Autodesk Inventor part; units mm, degrees
ref_plane "YZ Plane" through (0, 0, 0) normal (1, 0, 0) x (0, 1, 0)
ref_plane "XZ Plane" through (0, 0, 0) normal (0, 1, 0) x (-1, 0, 0)
ref_plane "XY Plane" through (0, 0, 0) normal (0, 0, 1) x (1, 0, 0)
sketch "Sketch1" plane through (0, 0, 0) normal (1, 0, 0) x (0, 1, 0)
  line L0 (0, 0) -> (-60, 0)
  line L1 (-60, 0) -> (-60, -18)
  line L2 (-60, -18) -> (0, -18)
  line L3 (0, -18) -> (0, 0)
  line L4 (-13.5, -5.5) -> (-33.5, -5.5)
  line L5 (-37, -9) -> (-37, -9)
  line L6 (-33.5, -12.5) -> (-13.5, -12.5)
  line L7 (-10, -9) -> (-10, -9)
  arc A0 (-10, -9) -> (-13.5, -5.5) centre (-13.5, -9) ccw
  arc A1 (-13.5, -12.5) -> (-10, -9) centre (-13.5, -9) ccw
  arc A2 (-37, -9) -> (-33.5, -12.5) centre (-33.5, -9) ccw
  arc A3 (-33.5, -5.5) -> (-37, -9) centre (-33.5, -9) ccw
  point P0 (-37, -12.5)
  point P1 (-37, -5.5)
  point P2 (-10, -12.5)
  dimension "d0" = 60
  dimension "d1" = 18
  dimension "d2" = 27
  dimension "d3" = 7
  dimension "d4" = 5.5
  dimension "d5" = 10
  dimension "d6" = 3.5
extrude "Extrusion1" add sketch "Sketch1" along normal blind 3
sketch "Sketch2" plane through (3, 0, 0) normal (1, 0, 0) x (0, 0, -1)
  line L0 (18, -60) -> (18, 0)
  line L1 (0, -60) -> (18, -60)
  point P0 (0, 0)
  point P1 (9, -45)
  point P2 (9, -55)
  dimension "d9" = 9
  dimension "d10" = 9
  dimension "d11" = 5
  dimension "d12" = 10
hole "Hole1" at (3, -45, -9) at (3, -55, -9) direction (-1, 0, 0) diameter 4.4 depth 8.8 tip angle 118
fillet "Fillet1" radius 3.5 2 edges at (1.5, -60, 0) (1.5, -60, -18)
chamfer "Chamfer1" distance 0.3 angle 45 25 edges at (3, 0, -9) (3, -28.25, -18) (3, -58.9749, -16.9749) (3, -60, -9) (3, -58.9749, -1.0251) (3, -28.25, 0) (1.5, 0, -18) (0, -28.25, -18) (0, -58.9749, -16.9749) (0, -60, -9) (0, -58.9749, -1.0251) (0, -28.25, 0) (0, 0, -9) (0, -10, -9) (0, -23.5, -5.5) (0, -37, -9) (0, -23.5, -12.5) (3, -23.5, -5.5) (3, -10, -9) (3, -23.5, -12.5) (3, -37, -9) (0, -55, -6.8) (0, -45, -6.8) (3, -55, -6.8) (3, -45, -6.8)
sketch "Sketch3" plane through (0, 0, 0) normal (-1, 0, 0) x (0, 0, 1)
  line L0 (-18, -0.3) -> (-18, -56.5)
  line L1 (0, -56.5) -> (0, 0)
  line L2 (0, 0) -> (-17.7, 0)
  point P0 (-15, -2)
  point P1 (-3, -2)
  dimension "d24" = 3
  dimension "d25" = 3
  dimension "d26" = 2
  dimension "d27" = 2
hole "Hole2" at (0, -2, -15) at (0, -2, -3) direction (1, 0, 0) diameter 2.4 depth 8.8 tip angle 118
properties part number "Ramka3" material "Steel"
Verification items for the finished model (mm, model axes). A direction names the side the tool comes from. Give positions to 0.01 mm unless a question says otherwise; leave off trailing zeros. Loops run counter-clockwise (first coordinate to the right, second up) from the corner with the lowest first, then second, coordinate; pieces in that order, holes last.
1) Thickness scan on line 1 along Y through (x, z) = (1.8, -9); line 2 along Z through (x, y) = (0.95, -31); line 3 along Y through (x, z) = (0.6, -7). Record the ranges inside material, lowest first.
2) Sectioned sample at B-B, the plane y = -30. Enter the section's corners in (x, z), then the cut area to 3 significant figures.
3) Set-up check for faces 1 (the flat face through (1, 0, -9)), 2 (the conical face through (0.18, -37.12, -9.08)), 3 (the conical face through (2.82, -9.88, -9.08)), 4 (the cylindrical face through (1, -37, -9)): record each of +Z, -Z, +X, -X, +Y, -Y from which the full face is reachable in a straight line by a thin tool's end or side.
4) Sectioned sample at D-D, the plane y = -45. Enter the section's corners in (x, z), then the cut area to 3 significant figures.
5) Sectioned sample at A-A, the plane y = -2. Enter the section's corners in (x, z).
6) Sectioned sample at C-C, the plane x = 2. Enter the section's corners in (y, z), then the cut area to 3 significant figures.
Answers:
1. line 1: y = -60 to -57.2, -52.8 to -47.2, -42.8 to -37, -10 to 0
1. line 2: z = -18 to -12.5, -5.5 to 0
1. line 3: y = -60 to -55.92, -54.08 to -45.92, -44.08 to -36.37, -10.63 to 0
2. outline: (0, -17.7) - (0.3, -18) - (2.7, -18) - (3, -17.7) - (3, -12.8) - (2.7, -12.5) - (0.3, -12.5) - (0, -12.8) - close; (0, -5.2) - (0.3, -5.5) - (2.7, -5.5) - (3, -5.2) - (3, -0.3) - (2.7, 0) - (0.3, 0) - (0, -0.3) - close
2. area: 32.6 mm2
3. face 1: +Z, -Z, +X, -X, +Y
3. face 2: -X
3. face 3: +X
3. face 4: +X, -X
4. outline: (0, -17.7) - (0.3, -18) - (2.7, -18) - (3, -17.7) - (3, -11.5) - (2.7, -11.2) - (0.3, -11.2) - (0, -11.5) - close; (0, -6.5) - (0.3, -6.8) - (2.7, -6.8) - (3, -6.5) - (3, -0.3) - (2.7, 0) - (0.3, 0) - (0, -0.3) - close
4. area: 40.4 mm2
5. outline: (0, -17.7) - (0.3, -18) - (2.7, -18) - (3, -17.7) - (3, -16.2) - (0, -16.2) - close; (0, -13.8) - (3, -13.8) - (3, -4.2) - (0, -4.2) - close; (0, -1.8) - (3, -1.8) - (3, -0.3) - (2.7, 0) - (0.3, 0) - (0, -0.3) - close
6. outline: (-60, -14.5) arc R3.5 ccw to (-56.5, -18) - (-0.3, -18) - (0, -17.7) - (0, 0) - (-56.5, 0) arc R3.5 ccw to (-60, -3.5) - close; hole circle Ø4.4 at (-55, -9); hole circle Ø4.4 at (-45, -9); hole (-33.5, -12.5) - (-13.5, -12.5) arc R3.5 ccw to (-13.5, -5.5) - (-33.5, -5.5) arc R3.5 ccw to start; hole circle Ø2.4 at (-2, -15); hole circle Ø2.4 at (-2, -3)
6. area: 857 mm2
